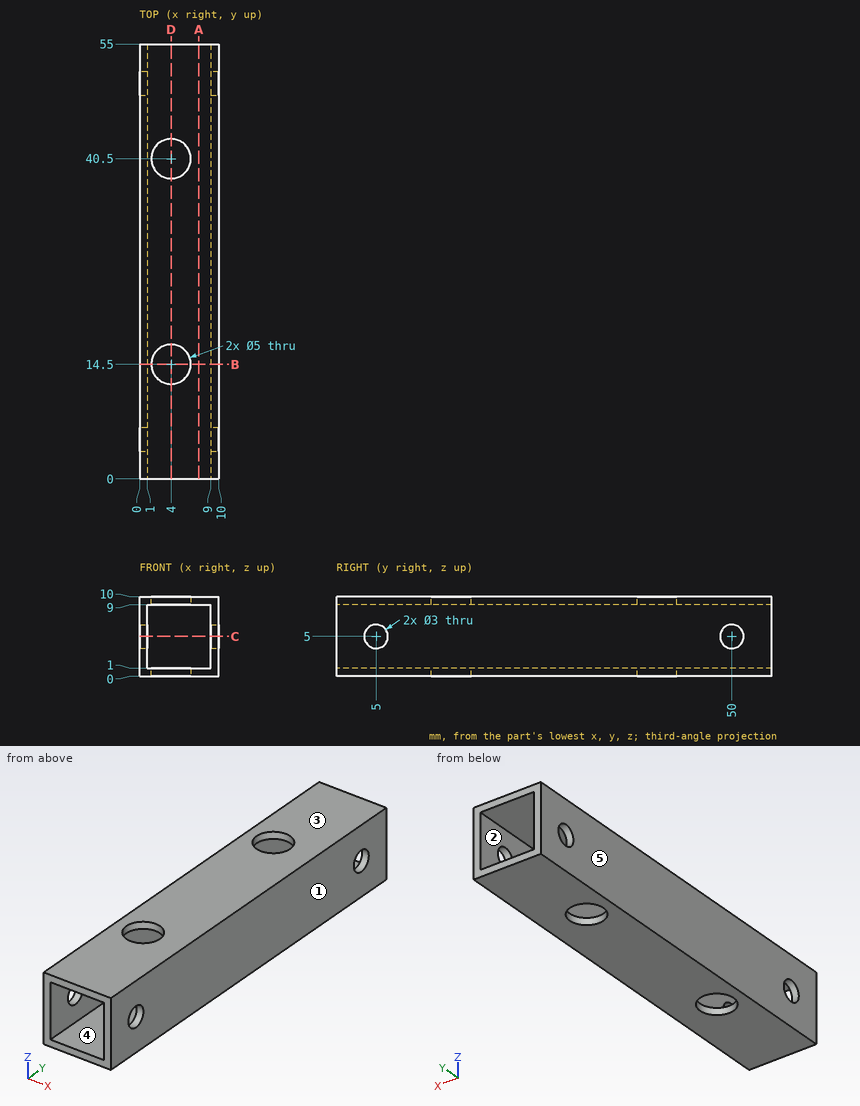
Could you check a few things on this drawing? It's one solid part, dimensions in mm from its lowest x, y, z. A direction names the side the tool comes from. Round coordinates to 2 decimals unless told otherwise and drop trailing zeros. Order: outer loops, then holes, each group sorted by start corner. A loop starts at its lowest first (then second) coordinate and runs counter-clockwise, first axis right, second up. Notation, with made-up numbers: (87.5, 21.25) -> (96.5, 21.25) arc R11 cw to (96.5, 28.25) -> close; hole circle Ø8 at (72, 17). An arc over 180 degrees is marked (long way). One line per question, with ' | ' between items.
Q1. If I drill on line 1 (Y direction, x = 4, z = 9.25); line 2 (Z direction, x = 9.65, y = 5); line 3 (Z direction, x = 4.25, y = 18.5), over which ranges is the centre line in solid material (lowest first)? Write a range as from..to.
Computed values:
line 1: 0..12, 17..38, 43..55 | line 2: 0..3.5, 6.5..10 | line 3: 0..1, 9..10
Q2. We'd pull the mould along Z, two halves only. Please class the marked faces 1, 2 and 3: released by +Z, released by -Z, zero draft, split by the parting line, or undercut.
Computed values:
face 1: zero draft | face 2: undercut | face 3: released by +Z
Q3. Which directions (+Z, -Z, +X, -X, +Y, -Y) give clear straight access to the entire face, cutting with the end or side of a thin tool? Please do the marked faces 4 and 5.
Computed values:
face 4: +Y, -Y | face 5: +Z, -Z, -X, +Y, -Y
Q4. If we section it at B-B on y = 14.5: Write out the boundary of the cut face in (x, z), plus the area to 3 significant figures.
Computed values:
outline: (0, 0) -> (1.5, 0) -> (1.5, 1) -> (1, 1) -> (1, 9) -> (1.5, 9) -> (1.5, 10) -> (0, 10) -> close; (6.5, 0) -> (10, 0) -> (10, 10) -> (6.5, 10) -> (6.5, 9) -> (9, 9) -> (9, 1) -> (6.5, 1) -> close | area: 26.0 mm²
Q5. I'm going to push flat-ended pins straight in: pin 1 (3 mm diameter, centred on y = 41.5, z = 7, fed in from -X); pin 2 (5 mm diameter, centred on x = 4, z = 5.5, fed in from -Y). Where does each tip first touch, or does it pass through?
Computed values:
pin 1: x = 0 | pin 2: through
Q6. If we section it at C-C on z = 5: Write out the boundary of the cut face in (x, y).
Computed values:
outline: (0, 0) -> (1, 0) -> (1, 3.5) -> (0, 3.5) -> close; (0, 6.5) -> (1, 6.5) -> (1, 48.5) -> (0, 48.5) -> close; (0, 51.5) -> (1, 51.5) -> (1, 55) -> (0, 55) -> close; (9, 0) -> (10, 0) -> (10, 3.5) -> (9, 3.5) -> close; (9, 6.5) -> (10, 6.5) -> (10, 48.5) -> (9, 48.5) -> close; (9, 51.5) -> (10, 51.5) -> (10, 55) -> (9, 55) -> close
Q7. If we section it at A-A on x = 7.5: Write out the boundary of the cut face in (y, z).
Computed values:
outline: (0, 0) -> (55, 0) -> (55, 1) -> (0, 1) -> close; (0, 9) -> (55, 9) -> (55, 10) -> (0, 10) -> close
Q8. If we section it at D-D on x = 4: Write out the boundary of the cut face in (y, z), plus the area to 3 significant figures.
Computed values:
outline: (0, 0) -> (12, 0) -> (12, 1) -> (0, 1) -> close; (0, 9) -> (12, 9) -> (12, 10) -> (0, 10) -> close; (17, 0) -> (38, 0) -> (38, 1) -> (17, 1) -> close; (17, 9) -> (38, 9) -> (38, 10) -> (17, 10) -> close; (43, 0) -> (55, 0) -> (55, 1) -> (43, 1) -> close; (43, 9) -> (55, 9) -> (55, 10) -> (43, 10) -> close | area: 90.0 mm²
